Job drawing, mm, ordinate dimensions from the low corner. One solid piece. Coordinates: 2 decimals unless noted, no trailing zeros. Write each loop counter-clockwise with the first axis right and the second up, starting at its lowest first coordinate (ties: lowest second). Pieces come first, ordered by that corner, then holes.
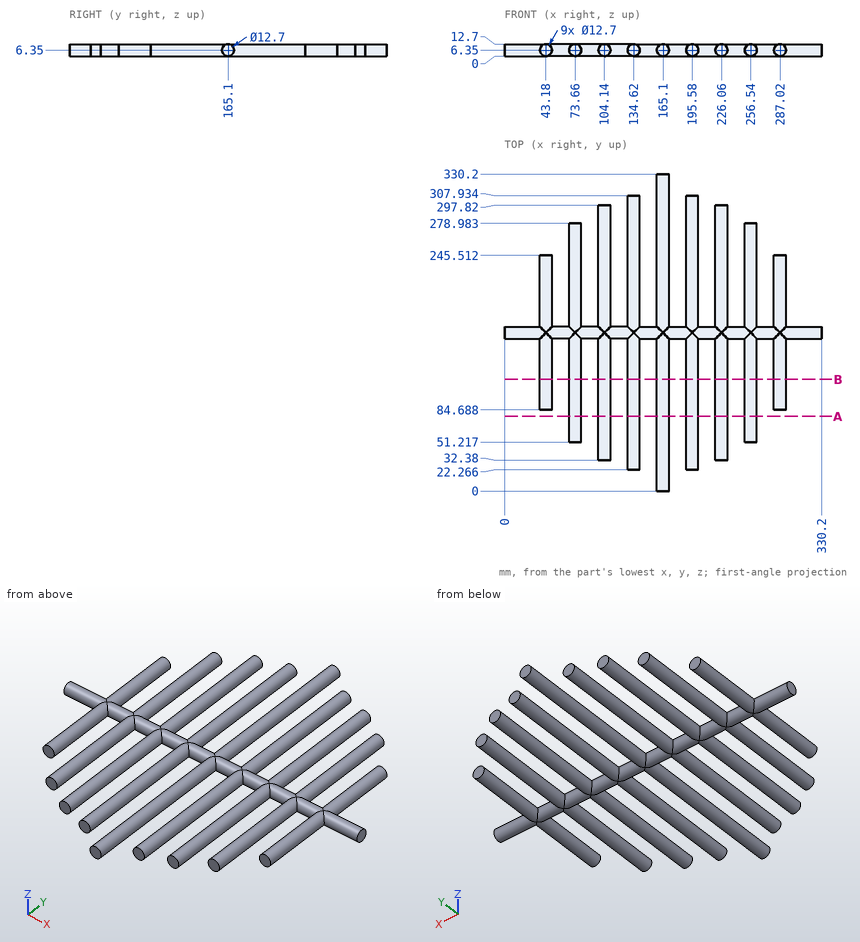
1. Saw through at B-B on y = 116.5. State how many separate pieces and enclosed holes the cut face has, plus the area to 3 significant figures.
Computed values:
separate pieces: 9
enclosed holes: 0
area: 1,140 mm2
2. Flat gauge pins, fed straight in: pin 1 (4 mm diameter, centred on x = 259.5, z = 5.5, fed in from -Y); pin 2 (6.5 mm diameter, centred on x = 105, z = 4.5, fed in from +Y); pin 3 (1.5 mm diameter, centred on x = 251.5, y = 247.5, fed in from -Z). Where does each tip first touch, or does it go through?
Computed values:
pin 1: stops at y = 51.22
pin 2: stops at y = 297.82
pin 3: stops at z = 1.67
3. Probe line 1 along X through (y, z) = (282, 11.5) (1 decimal); line 2 along Y through (x, z) = (261, 4.25); line 3 along Y through (x, z) = (225.5, 5.25). List the from-to ranges inside material, lowest first.
Computed values:
line 1: x = 100.4 to 107.9, 130.9 to 138.3, 161.4 to 168.8, 191.9 to 199.3, 222.3 to 229.8
line 2: y = 51.22 to 278.98
line 3: y = 32.38 to 297.82
4. Saw through at A-A on y = 78. List the corners of the cut face in (x, z).
Computed values:
outline: circle Ø12.7 at (73.66, 6.35); circle Ø12.7 at (104.14, 6.35); circle Ø12.7 at (134.62, 6.35); circle Ø12.7 at (165.1, 6.35); circle Ø12.7 at (195.58, 6.35); circle Ø12.7 at (226.06, 6.35); circle Ø12.7 at (256.54, 6.35)
